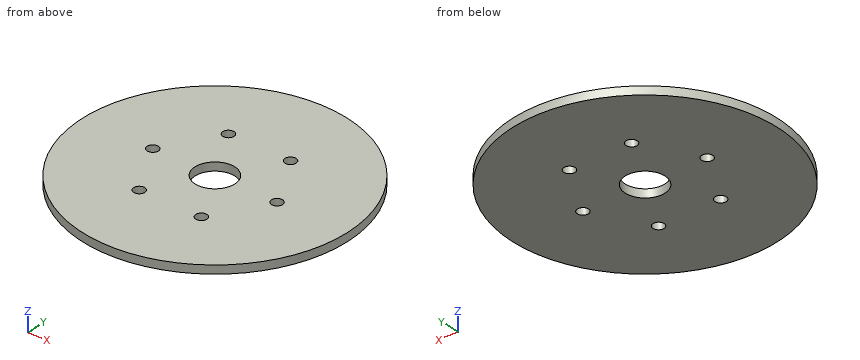
Autodesk Inventor part; units mm, degrees
ref_plane "YZ Plane" through (0, 0, 0) normal (1, 0, 0) x (0, 1, 0)
ref_plane "XZ Plane" through (0, 0, 0) normal (0, 1, 0) x (-1, 0, 0)
ref_plane "XY Plane" through (0, 0, 0) normal (0, 0, 1) x (1, 0, 0)
sketch "Sketch1" plane through (0, 0, 0) normal (0, 0, 1) x (1, 0, 0)
  circle A0 centre (23.8125, 0) radius 2.1463
  circle A1 centre (11.9063, 20.6222) radius 2.1463
  circle A2 centre (-11.9062, 20.6222) radius 2.1463
  circle A3 centre (-23.8125, 0) radius 2.1463
  circle A4 centre (-11.9063, -20.6222) radius 2.1463
  circle A5 centre (11.9062, -20.6222) radius 2.1463
  circle A6 centre (0, 0) radius 50.8
  circle A7 centre (0, 0) radius 7.62
  dimension "d0" = 4.2926
  dimension "d4" = 360
  dimension "d6" = 101.6
  dimension "d9" = 15.24
extrude "Extrusion1" add sketch "Sketch1" along normal mid plane 3.175
properties part number "Spool Plate" material "Aluminum 6061"
Can you work these out from the model? Positions are in its coordinate system, mm. Round coordinates to 2 decimals unless told otherwise and drop trailing zeros. Loops run counter-clockwise (first coordinate to the right, second up) from the corner with the lowest first, then second, coordinate; pieces in that order, holes last. Notation, with made-up numbers: (13.25, -8) - (56.25, -8) arc R27 ccw to (56.25, 28) - close; hole circle Ø11 at (-30.75, 28). An arc over 180 degrees is marked (long way). Answer in a Markdown table with one row per item. Add a question column.
Q1. I need wall thicknesses on L1, parallel to X at y = 19, z = 1.3; L2, parallel to Y at x = 0, z = -1; L3, parallel to X at y = -5.5, z = 1.4. Which ranges of each line are inside material? Lowest first, please.
Q2. For pin 1 Ø2.5 at (x, y) = (11.91, -20.62) entering from +Z; pin 2 Ø1 at (x, z) = (-35, 0.5) entering from -Y, each with a flat end and sliding along its axis, tell me the tip position at first contact or that it passes through.
Q3. I want a section at B-B on x = 0. List the corners of the cut face in (y, z) for me.
Q4. I want a section at D-D on z = -0.45. List the corners of the cut face in (x, y) for me.
Q5. I want a section at C-C on x = 11. List the corners of the cut face in (y, z) for me.
Q6. I want a section at A-A on y = 0. List the corners of the cut face in (x, z) for me.
A:
| question | item | result |
|---|---|---|
| 1 | L1 | -47.11 to -13.31, -10.5 to 10.5, 13.31 to 47.11 |
| 1 | L2 | -50.8 to -7.62, 7.62 to 50.8 |
| 1 | L3 | -50.5 to -5.27, 5.27 to 50.5 |
| 2 | pin 1 | through |
| 2 | pin 2 | y = -37.29 |
| 3 | outline | (-50.8, -1.59) - (-7.62, -1.59) - (-7.62, 1.59) - (-50.8, 1.59) - close; (7.62, -1.59) - (50.8, -1.59) - (50.8, 1.59) - (7.62, 1.59) - close |
| 4 | outline | circle Ø101.6 at (0, 0); hole circle Ø4.29 at (-23.81, 0); hole circle Ø4.29 at (-11.91, -20.62); hole circle Ø4.29 at (-11.91, 20.62); hole circle Ø15.24 at (0, 0); hole circle Ø4.29 at (11.91, -20.62); hole circle Ø4.29 at (11.91, 20.62); hole circle Ø4.29 at (23.81, 0) |
| 5 | outline | (-49.59, -1.59) - (-22.57, -1.59) - (-22.57, 1.59) - (-49.59, 1.59) - close; (-18.68, -1.59) - (18.68, -1.59) - (18.68, 1.59) - (-18.68, 1.59) - close; (22.57, -1.59) - (49.59, -1.59) - (49.59, 1.59) - (22.57, 1.59) - close |
| 6 | outline | (-50.8, -1.59) - (-25.96, -1.59) - (-25.96, 1.59) - (-50.8, 1.59) - close; (-21.67, -1.59) - (-7.62, -1.59) - (-7.62, 1.59) - (-21.67, 1.59) - close; (7.62, -1.59) - (21.67, -1.59) - (21.67, 1.59) - (7.62, 1.59) - close; (25.96, -1.59) - (50.8, -1.59) - (50.8, 1.59) - (25.96, 1.59) - close |
